```python
from build123d import *

# Parameters (mm, degrees)
SKETCH_W        = 13
SKETCH_H        = 8.2
PAD_DEPTH       = 8.3
SKETCH001_W     = 15.1
SKETCH001_H     = 10.5
PAD001_DEPTH    = 1.4
CHAMFER_SIZE    = 1
PAD002_DEPTH    = 3
FILLET_R        = 1
SKETCH003_W     = 0.33
SKETCH003_H     = 3.7
PAD003_DEPTH    = 6.65
CHAMFER001_SIZE = 1.5


with BuildPart() as part:
    # Sketch → Pad (new body)
    with BuildSketch(Plane.XY):
        Rectangle(SKETCH_W, SKETCH_H)
    extrude(amount=-PAD_DEPTH)

    # Sketch001 → Pad001 (join)
    with BuildSketch(Plane.XY):
        Rectangle(SKETCH001_W, SKETCH001_H)
    extrude(amount=PAD001_DEPTH)

    # Chamfer
    chamfer_edges = [part.edges().sort_by_distance(p)[0] for p in [
        (-7.55, 0, 1.4),
        (0, 5.25, 1.4),
        (7.55, 0, 1.4),
        (0, -5.25, 1.4),
    ]]
    chamfer(chamfer_edges, length=CHAMFER_SIZE)

    # Sketch002 → Pad002 (join, symmetric)
    with BuildSketch(Plane.XZ):
        with BuildLine():
            Line((-5.5, 1.4), (5.5, 1.4))
            ThreePointArc((5.5, 1.4), (4.48879, 3.316002), (2.739315, 4.593869))
            ThreePointArc((-5.5, 1.4), (-1.081654, 2.2264), (2.739315, 4.593869))
        make_face()
    extrude(amount=PAD002_DEPTH, both=True)

    # Fillet
    fillet_edges = [part.edges().sort_by_distance(p)[0] for p in [
        (2.739315, 0, 4.593869),
    ]]
    fillet(fillet_edges, radius=FILLET_R)

    # Sketch003 (on DatumPlane) → Pad003 (join)
    with BuildSketch(Plane.XY.offset(-8.3)):
        with Locations((4.035, 0)):
            Rectangle(SKETCH003_W, SKETCH003_H)
        with Locations((-0.895, 0)):
            Rectangle(SKETCH003_W, SKETCH003_H)
    extrude(amount=-PAD003_DEPTH)

    # Chamfer001
    chamfer001_edges = [part.edges().sort_by_distance(p)[0] for p in [
        (4.035, 1.85, -14.95),
        (4.035, -1.85, -14.95),
        (-0.895, 1.85, -14.95),
        (-0.895, -1.85, -14.95),
    ]]
    chamfer(chamfer001_edges, length=CHAMFER001_SIZE)


solid = part.part
```
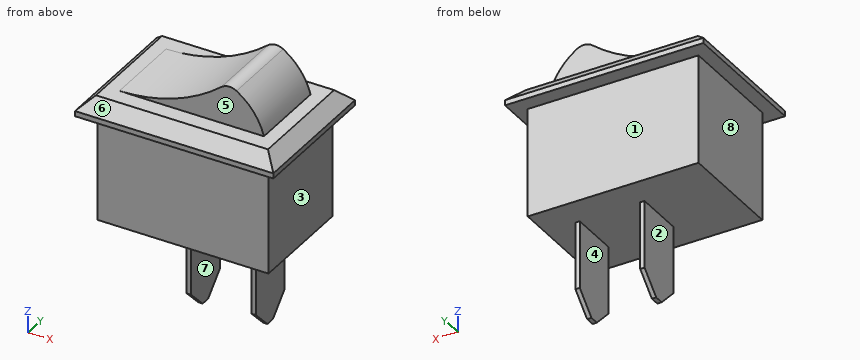
Input: part model. Units: mm. Frame: model coordinates. Face numbers are marked on the shaded views. A direction names the side the tool comes from. Coordinates: 2 decimals unless noted, no trailing zeros. Write each loop counter-clockwise with the first axis right and the second up, starting at its lowest first coordinate (ties: lowest second). Pieces come first, ordered by that corner, then holes. Notation, with made-up numbers: M 43.5,69 L 56.5,69 A19 cw 56.5,75 Z; hole C 47,67.25 d8. An arc over 180 degrees is marked long. Use one line per item in the form item = value.
Q1. Section C-C (x = 5.75). Return loops of the section in (y, z), plus the area to 3 significant figures.
Answer below:
outline = M -5.25,0 L -4.1,0 L -4.1,-8.3 L 4.1,-8.3 L 4.1,0 L 5.25,0 L 5.25,0.4 L 4.25,1.4 L -4.25,1.4 L -5.25,0.4 Z
area = 81.8 mm²
Q2. Section B-B (y = -3.75). Return loops of the section in (x, z).
Answer below:
outline = M -7.55,0 L -6.5,0 L -6.5,-8.3 L 6.5,-8.3 L 6.5,0 L 7.55,0 L 7.55,0.4 L 6.55,1.4 L -6.55,1.4 L -7.55,0.4 Z
Q3. Set-up query: the marked faces 1, 2, 3, 4 and 5. Return all of +Z, -Z, +X, -X, +Y, -Y with unobstructed straight access to the full face (end or side cutting, diameter ignored); none if empty.
Answer below:
face_1 = -Z, +X, -X, +Y
face_2 = -Z, -X, +Y, -Y
face_3 = -Z, +X, +Y, -Y
face_4 = -Z, +Y, -Y
face_5 = +Z, +X, -X, -Y
Q4. Section D-D (z = -6.5). Return loops of the section in (x, y), plus the area to 3 significant figures.
Answer below:
outline = M -6.5,-4.1 L 6.5,-4.1 L 6.5,4.1 L -6.5,4.1 Z
area = 107 mm²
Q5. First-contact query: pin 1 (2.5 mm diameter, centred on y = 0, z = -3.5, fed in from -X); pin 2 (2.5 mm diameter, centred on x = 2, z = 3, fed in from -Y); pin 3 (2.5 mm diameter, centred on x = -2, z = -4, fed in from +Y); pin 4 (0.9 mm diameter, centred on x = -2.5, z = 3, fed in from +Y). Flat tips, straight axial feed; report the tip coordinate or a pass-through.
Answer below:
pin_1 = -6.5
pin_2 = -3
pin_3 = 4.1
pin_4 = through
Q6. Section A-A (z = -11.5). Return loops of the section in (x, y), plus the area to 3 significant figures.
Answer below:
outline = M -1.06,-1.85 L -0.73,-1.85 L -0.73,1.85 L -1.06,1.85 Z; M 3.87,-1.85 L 4.2,-1.85 L 4.2,1.85 L 3.87,1.85 Z
area = 2.44 mm²
Q7. Draft query along X for the marked faces 6, 7 and 8. Return one class per face: released by +X, released by -X, zero draft, split by the parting line, or undercut.
Answer below:
face_6 = zero draft
face_7 = undercut
face_8 = released by -X
Q8. Material intervals for probe 1 along X at (y, z) = (0.5, -11.25); probe 2 along X at (y, z) = (2.25, -4.5); probe 3 along Z at (x, y) = (-3.75, -4), sorted ascending. Write a range as from..to.
Answer below:
probe_1 = -1.06..-0.73, 3.87..4.2
probe_2 = -6.5..6.5
probe_3 = -8.3..1.4
